from build123d import *

# Parameters (mm, degrees)
SKETCH1_R           = 7.472749452
BOSS_EXTRUDE1_DEPTH = 25.4
SKETCH2_W           = 14.945498904
SKETCH2_H           = 22.418248356
BOSS_EXTRUDE2_DEPTH = 0.863350236
SKETCH4_W           = 63.40856
SKETCH4_H           = 4.26981756
BOSS_EXTRUDE3_DEPTH = 27.00421054
SKETCH6_W           = 27.00421054
SKETCH6_H           = 4.26981756
BOSS_EXTRUDE4_DEPTH = 0.56888896
SKETCH7_W           = 0.56888896
SKETCH7_H           = 27.00421054
BOSS_EXTRUDE5_DEPTH = 38.0746
SKETCH8_W           = 0.56888896
SKETCH8_H           = 27.00421054
BOSS_EXTRUDE6_DEPTH = 0.853447309
SKETCH9_W           = 27.00421054
SKETCH9_H           = 0.853447309
BOSS_EXTRUDE7_DEPTH = 25.37968
MIRROR1_START       = -32.27316896
MIRROR1_OUTLINE_W   = 43.197864869
MIRROR1_OUTLINE_H   = 27.00421054
MIRROR1_DEPTH       = 0.56888896
MIRROR1_START_2     = -31.70428
MIRROR1_2_OUTLINE_W = 0.853447309
MIRROR1_2_OUTLINE_H = 27.00421054
MIRROR1_2_DEPTH     = 25.37968


# Read off the part's stored shape, not the designer's step: Mirror1
with BuildPart() as part:
    # Sketch1 → Boss-Extrude1 (new body)
    with BuildSketch(Plane.XY):
        Circle(SKETCH1_R)
    extrude(amount=-BOSS_EXTRUDE1_DEPTH)

    # Sketch2 → Boss-Extrude2 (add)
    with BuildSketch(Plane(origin=(0, 0, -25.4), x_dir=(-1, 0, 0), z_dir=(0, 0, -1))):
        with BuildLine():
            ThreePointArc((7.472749452, 0), (0, 7.472749452), (-7.472749452, 0))
            Line((-7.472749452, 0), (7.472749452, 0))
        make_face()
        with BuildLine():
            Line((7.472749452, 0), (-7.472749452, 0))
            ThreePointArc((-7.472749452, 0), (0, -7.472749452), (7.472749452, 0))
        make_face()
        with BuildLine():
            ThreePointArc((7.472749452, 0), (0, 7.472749452), (-7.472749452, 0))
            Line((-7.472749452, 0), (7.472749452, 0))
        make_face()
        with BuildLine():
            Line((7.472749452, 0), (-7.472749452, 0))
            ThreePointArc((-7.472749452, 0), (0, -7.472749452), (7.472749452, 0))
        make_face()
        with Locations((0, 11.209124178)):
            Rectangle(SKETCH2_W, SKETCH2_H)
    extrude(amount=BOSS_EXTRUDE2_DEPTH)

    # Sketch4 → Boss-Extrude3 (add)
    with BuildSketch(Plane(origin=(0, 0, -26.263350236), x_dir=(-1, 0, 0), z_dir=(0, 0, -1))):
        with Locations((0, 24.553157136)):
            Rectangle(SKETCH4_W, SKETCH4_H)
    extrude(amount=-BOSS_EXTRUDE3_DEPTH)

    # Sketch6 → Boss-Extrude4 (add)
    with BuildSketch(Plane(origin=(31.70428, 0, 0), x_dir=(0, 0, -1), z_dir=(1, 0, 0))):
        with Locations((12.761244966, 24.553157136)):
            Rectangle(SKETCH6_W, SKETCH6_H)
    extrude(amount=BOSS_EXTRUDE4_DEPTH)

    # Sketch7 → Boss-Extrude5 (add)
    with BuildSketch(Plane(origin=(0, 26.688065916, 0), x_dir=(1, 0, 0), z_dir=(0, 1, 0))):
        with Locations((31.98872448, 12.761244966)):
            Rectangle(SKETCH7_W, SKETCH7_H)
    extrude(amount=BOSS_EXTRUDE5_DEPTH)

    # Sketch8 → Boss-Extrude6 (add)
    with BuildSketch(Plane(origin=(0, 64.762665916, 0), x_dir=(1, 0, 0), z_dir=(0, 1, 0))):
        with Locations((31.98872448, 12.761244966)):
            Rectangle(SKETCH8_W, SKETCH8_H)
    extrude(amount=BOSS_EXTRUDE6_DEPTH)

    # Sketch9 → Boss-Extrude7 (add)
    with BuildSketch(Plane.ZY.offset(-31.70428)):
        with Locations((-12.761244966, 65.18938957)):
            Rectangle(SKETCH9_W, SKETCH9_H)
    extrude(amount=BOSS_EXTRUDE7_DEPTH)

    # Mirror1 outline → Mirror1 (add)
    with BuildSketch(Plane.YZ.offset(MIRROR1_START)):
        with Locations((44.017180791, -12.761244966)):
            Rectangle(MIRROR1_OUTLINE_W, MIRROR1_OUTLINE_H)
    extrude(amount=MIRROR1_DEPTH)

    # Mirror1 2 outline → Mirror1 2 (add)
    with BuildSketch(Plane.YZ.offset(MIRROR1_START_2)):
        with Locations((65.18938957, -12.761244966)):
            Rectangle(MIRROR1_2_OUTLINE_W, MIRROR1_2_OUTLINE_H)
    extrude(amount=MIRROR1_2_DEPTH)


solid = part.part
Could you check a few things on this model? Use its own coordinates, in mm. A direction names the side the tool comes from. Give positions to 0.01 mm unless a question says otherwise; leave off trailing zeros. Loops run counter-clockwise (first coordinate to the right, second up) from the corner with the lowest first, then second, coordinate; pieces in that order, holes last. Notation, with made-up numbers: (70, 14) -> (96, 14) arc R15 ccw to (96, 25) -> close; hole circle Ø10 at (43, 44). An arc over 180 degrees is marked (long way). Answer as CSV lines item,"result". Start each with the question number.
(1) If we section it at D-D on x = 0: Write out the boundary of the cut face in (y, z), then the cut area to 3 significant figures.
(2) I need wall thicknesses on probe 1 along Y at (x, z) = (19, -5.5); probe 2 along X at (y, z) = (28.5, -10.5); probe 3 along Y at (x, z) = (6, -12). Which ranges of each line are inside material? Lowest first, please.
(3) If we section it at B-B on x = -21.5: Write out the boundary of the cut face in (y, z).
(4) If we section it at A-A on y = 49.5: Write out the boundary of the cut face in (x, z).
(5) Which directions (+Z, -Z, +X, -X, +Y, -Y) give clear straight access to the entire face, cutting with the end or side of a thin tool? Please do faces 5 (the flat face through (0, 25, 0.741)), 6 (the flat face through (31.704, 45, -13)), 7 (the flat face through (0, 0, 0)).
(6) We'd pull the mould along X, two halves only. Please class faces 1 (the flat face through (32.273, 44, -13)), 2 (the flat face through (19, 64.763, -13)), 3 (the flat face through (19, 65.616, -13)), 4 (the flat face through (-32.273, 44, -13)): released by +X, released by -X, zero draft, split by the parting line, or undercut.
(7) I'm going to push flat-ended pins straight in: pin 1 Ø4 at (y, z) = (8, -11.5) entering from +X; pin 2 Ø1 at (x, y) = (-8.5, 16) entering from -Z; pin 3 Ø13.5 at (x, z) = (5.5, -16) entering from -Y; pin 4 Ø0.9 at (y, z) = (10.5, -25.5) entering from +X. Where does each tip first touch, or does it pass through?
(8) If we section it at C-C on z = -15.25: Write out the boundary of the cut face in (x, y), then the cut area to 3 significant figures.
Computed:
1,outline,"(-7.47, -26.26) -> (26.69, -26.26) -> (26.69, 0.74) -> (22.42, 0.74) -> (22.42, -25.4) -> (7.47, -25.4) -> (7.47, 0) -> (-7.47, 0) -> close"
1,area,"521 mm2"
2,probe 1,"y = 22.42 to 26.69, 64.76 to 65.62"
2,probe 2,"x = -32.27 to -31.7, 31.7 to 32.27"
2,probe 3,"y = -4.45 to 4.45, 22.42 to 26.69"
3,outline,"(22.42, -26.26) -> (26.69, -26.26) -> (26.69, 0.74) -> (22.42, 0.74) -> close; (64.76, -26.26) -> (65.62, -26.26) -> (65.62, 0.74) -> (64.76, 0.74) -> close"
4,outline,"(-32.27, -26.26) -> (-31.7, -26.26) -> (-31.7, 0.74) -> (-32.27, 0.74) -> close; (31.7, -26.26) -> (32.27, -26.26) -> (32.27, 0.74) -> (31.7, 0.74) -> close"
5,face 5,"+Z, +X, -X, +Y, -Y"
5,face 6,"+Z, -Z"
5,face 7,"+Z, +X, -X, -Y"
6,face 1,"released by +X"
6,face 2,"undercut"
6,face 3,"zero draft"
6,face 4,"released by -X"
7,pin 1,"stops at x = 4.45"
7,pin 2,"passes through"
7,pin 3,"stops at y = -7.47"
7,pin 4,"stops at x = 7.47"
8,outline,"(-32.27, 22.42) -> (32.27, 22.42) -> (32.27, 65.62) -> (6.32, 65.62) -> (6.32, 64.76) -> (31.7, 64.76) -> (31.7, 26.69) -> (-31.7, 26.69) -> (-31.7, 64.76) -> (-6.32, 64.76) -> (-6.32, 65.62) -> (-32.27, 65.62) -> close; circle Ø14.95 at (0, 0)"
8,area,"539 mm2"
